Part model, mm, in its own coordinate system. A direction names the side the tool comes from. Round coordinates to 2 decimals unless told otherwise and drop trailing zeros. Write each loop counter-clockwise with the first axis right and the second up, starting at its lowest first coordinate (ties: lowest second). Pieces come first, ordered by that corner, then holes.
```python
from build123d import *

# Parameters (mm, degrees)
SKETCH_W     = 91
SKETCH_H     = 91
PAD_DEPTH    = 29
SKETCH001_W  = 84.1
SKETCH001_H  = 84.1
POCKET_DEPTH = 26


with BuildPart() as part:
    # Sketch (on XZ_Plane of Origin) → Pad (new body)
    with BuildSketch(Plane.XZ):
        Rectangle(SKETCH_W, SKETCH_H)
    extrude(amount=PAD_DEPTH)

    # Sketch001 (on XZ_Plane of Origin) → Pocket (cut)
    with BuildSketch(Plane.XZ):
        Rectangle(SKETCH001_W, SKETCH001_H)
    extrude(amount=POCKET_DEPTH, mode=Mode.SUBTRACT)


solid = part.part
```
Q1. Which spindle directions (+Z, -Z, +X, -X, +Y, -Y) get a long thin tool onto all of the face, cutting with end or side? Do faces 1 (the flat face through (-1, -29, 1)), 2 (the flat face through (-1, -26, 1)). Say none if no direction does.
Values follow:
face 1: +Z, -Z, +X, -X, -Y
face 2: +Y
Q2. Wall check: L1, parallel to X at y = -18.5, z = -16; L2, parallel to Y at x = 41, z = -29.5. Give the ranges that are in metal, low to high.
Values follow:
L1: x = -45.5 to -42.05, 42.05 to 45.5
L2: y = -29 to -26
Q3. Cut at A-A on y = -18.5. Write the cut outline in (x, z).
Values follow:
outline: (-45.5, -45.5) - (45.5, -45.5) - (45.5, 45.5) - (-45.5, 45.5) - close; hole (-42.05, -42.05) - (42.05, -42.05) - (42.05, 42.05) - (-42.05, 42.05) - close
Q4. Cut at C-C on x = 22.5. Write the cut outline in (y, z), plus the area to 3 significant figures.
Values follow:
outline: (-29, -45.5) - (0, -45.5) - (0, -42.05) - (-26, -42.05) - (-26, 42.05) - (0, 42.05) - (0, 45.5) - (-29, 45.5) - close
area: 452 mm2
Q5. Drop a flat-ended pin along its axis: pin 1 (10 mm diameter, centred on x = -36, z = 14.5, fed in from +Y). Give the stop position or say it passes through.
Values follow:
pin 1: stops at y = -26
Q6. Cut at B-B on z = 4. Write the cut outline in (x, y), plus the area to 3 significant figures.
Values follow:
outline: (-45.5, -29) - (45.5, -29) - (45.5, 0) - (42.05, 0) - (42.05, -26) - (-42.05, -26) - (-42.05, 0) - (-45.5, 0) - close
area: 452 mm2
Q7. Mould opens along X. For faces 3 (the flat face through (-42.05, -13, -1)), 4 (the flat face through (-45.5, -14, -1)), 5 (the flat face through (45.5, -14, -1)), 6 (the flat face through (-1, -14, -45.5)) say: +X half, -X half, draft (parallel to the pull), parting line (faces both ways), or undercut.
Values follow:
face 3: undercut
face 4: -X half
face 5: +X half
face 6: draft
